```python
from build123d import *

# Parameters (mm, degrees)
F0_R     = 3.27
F1_DEPTH = 5.87
F2_R     = 3.15
F3_W     = 12.847729
F3_H     = 2.14129
F4_DEPTH = 3.01
F5_R     = 1.353715
F6_DEPTH = 25.4
F7_R     = 2.551292
F8_DEPTH = 3.54


with BuildPart() as f1:
    # F0 (on Front) → F1 (new body)
    with BuildSketch(Plane.XZ):
        with Locations((-25.3723, 25.103809)):
            Circle(F0_R)
    extrude(amount=F1_DEPTH)

    # F2
    f2_edges = [f1.edges().sort_by_distance(p)[0] for p in [
        (-28.6423, -5.87, 25.103809),
    ]]
    fillet(f2_edges, radius=F2_R)

    # F3 (on face) → F4 (cut)
    with BuildSketch(Plane.XZ.offset(5.87)):
        with Locations((-25.525428, 25.025891)):
            Rectangle(F3_W, F3_H)
    extrude(amount=-F4_DEPTH, mode=Mode.SUBTRACT)

    # F5 (on Front) → F6 (cut)
    with BuildSketch(Plane.XZ):
        with Locations((-25.255676, 25.105048)):
            Circle(F5_R)
    extrude(amount=F6_DEPTH, mode=Mode.SUBTRACT)

    # F7 (on Front) → F8 (cut)
    with BuildSketch(Plane.XZ):
        with Locations((-25.405101, 25.131198)):
            Circle(F7_R)
    extrude(amount=F8_DEPTH, mode=Mode.SUBTRACT)


solid = f1.part
```
Verification items for the finished model (mm, model axes). A direction names the side the tool comes from. Round coordinates to 2 decimals unless told otherwise and drop trailing zeros. Write each loop counter-clockwise with the first axis right and the second up, starting at its lowest first coordinate (ties: lowest second). Pieces come first, ordered by that corner, then holes.
1. Section check A-A on y = -0.65. Enter the section's corners in (x, z), plus the area to 3 significant figures.
2. Access from +Z, -Z, +X, -X, +Y, -Y to the whole of each face (thin tool, end or side, straight path). Record for faces 1 (the cylindrical face through (-25.24, -4.58, 26.46)), 2 (the cylindrical face through (-27.954, -1.745, 25.243)), 3 (the flat face through (-24, -4, 26.097)).
3. Gauge pin test, flat ends, axial feed: P1, Ø1.1, axis at x = -28, z = 25, coming from the -Y side; P2, Ø1.1, axis at x = -23, y = -4.5, coming from the +Z side; P3, Ø1.2, axis at x = -27, y = -5, coming from the -Z side. Record the tip position at first contact, or that the pin passes through.
4. Scan lines: L1, parallel to Z at x = -27.5, y = -1.35 (3 decimals); L2, parallel to Z at x = -26, y = -0.35; L3, parallel to X at y = -1.65, z = 25.75. Record each from-to range of solid material in increasing order.
5. Draft check along Z on faces 4 (the cylindrical face through (-25.27, -4.58, 23.75)), 5 (the cylindrical face through (-27.782, -1.341, 27.314)). Enter one of: +Z half, -Z half, draft (parallel to the pull), parting line (faces both ways), or undercut.
Answer:
1. outline: circle Ø6.54 at (-25.37, 25.1); hole circle Ø5.1 at (-25.41, 25.13)
1. area: 13.1 mm2
2. face 1: +Y, -Y
2. face 2: +Y
2. face 3: +X, -X, -Y
3. P1: stops at y = -2.86
3. P2: stops at z = 27.29
3. P3: stops at z = 22.71
4. L1: z = 22.621 to 23.675, 26.587 to 27.587
4. L2: z = 21.89 to 22.65, 27.61 to 28.31
4. L3: x = -28.58 to -27.88, -22.93 to -22.17
5. face 4: undercut
5. face 5: parting line
